```python
from build123d import *

# Parameters (mm, degrees)
F2_DEPTH = 7.5


with BuildPart() as f1:
    # F0 (on Front) → F1 (revolve)
    with BuildSketch(Plane.XZ):
        with BuildLine():
            Line((16.234176, 0), (0, 0))
            Line((0, 0), (0, -18.89116))
            Line((0, -18.89116), (14.934336, -18.89116))
            ThreePointArc((14.934336, -18.89116), (14.908992, -14.946672), (16.234176, -11.231363))
            ThreePointArc((16.234176, -11.231363), (14.748893, -5.615682), (16.234176, 0))
        make_face()
    revolve(axis=Axis((0, 0, -9.44558), (0, 0, 1)))

    # F0 (on Front) → F2 (join, symmetric)
    with BuildSketch(Plane.XZ):
        Polygon((-16.234176, 0), (0, 0), (16.234176, 0), (50.981011, 61.091773), (0, 34.319621), (-50.981011, 61.091773), align=None)
        with BuildLine():
            Line((16.234176, 0), (0, 0))
            Line((0, 0), (0, -18.89116))
            Line((0, -18.89116), (14.934336, -18.89116))
            ThreePointArc((14.934336, -18.89116), (14.908992, -14.946672), (16.234176, -11.231363))
            ThreePointArc((16.234176, -11.231363), (14.748893, -5.615682), (16.234176, 0))
        make_face()
    extrude(amount=F2_DEPTH, both=True)


solid = f1.part
```
Verification items for the finished model (mm, model axes). A direction names the side the tool comes from. Coordinates: 2 decimals unless noted, no trailing zeros. Write each loop counter-clockwise with the first axis right and the second up, starting at its lowest first coordinate (ties: lowest second). Pieces come first, ordered by that corner, then holes. Notation, with made-up numbers: (-39, 4.5) - (-4, 4.5) arc R28 cw to (-4, 30.5) - close; hole circle Ø7 at (26, 19.25). An arc over 180 degrees is marked (long way). Write item = value, one per line.
Q1. Mould release check, pull along Z, two halves, no side actions. Record for faces 1 (the face through (33.364, -0.105, 30.118)), 2 (the face through (25.847, -0.105, 47.893)), 3 (the face through (14.9, -0.1, -15)): released by +Z, released by -Z, zero draft, split by the parting line, or undercut.
Answer:
face_1 = released by -Z
face_2 = released by +Z
face_3 = undercut
Q2. Material ranges on L1, parallel to Y at x = -3, z = 19; L2, parallel to X at y = -3, z = 55; L3, parallel to Z at x = 10.5, y = 8, recorded low to high. Write a range as from..to.
Answer:
L1 = -7.5..7.5
L2 = -47.52..-39.38, 39.38..47.52
L3 = -18.89..0
Q3. Access from +Z, -Z, +X, -X, +Y, -Y to the whole of each face (thin tool, end or side, straight path). Record for faces 4 (the face through (0, 11, 0)), 5 (the face through (0, -11, 0)), 6 (the face through (-25.1, -0.1, 47.5)), 7 (the face through (-33.85, -0.11, 30.97)).
Answer:
face_4 = +Z, +X, -X, +Y
face_5 = +Z, +X, -X, -Y
face_6 = +Z, +Y, -Y
face_7 = -Z, -X, +Y, -Y
Q4. Cross-section at B-B (x = 37). Enter the section's corners in (y, z).
Answer:
outline = (-7.5, 36.51) - (7.5, 36.51) - (7.5, 53.75) - (-7.5, 53.75) - close
Q5. Cross-section at C-C (z = 43.5). Enter the section's corners in (x, y).
Answer:
outline = (-40.98, -7.5) - (-17.48, -7.5) - (-17.48, 7.5) - (-40.98, 7.5) - close; (17.48, -7.5) - (40.98, -7.5) - (40.98, 7.5) - (17.48, 7.5) - close
Q6. Cross-section at A-A (z = 35.5). Enter the section's corners in (x, y), plus the area to 3 significant figures.
Answer:
outline = (-36.43, -7.5) - (-2.25, -7.5) - (-2.25, 7.5) - (-36.43, 7.5) - close; (2.25, -7.5) - (36.43, -7.5) - (36.43, 7.5) - (2.25, 7.5) - close
area = 1,030 mm²
Q7. Cross-section at D-D (z = -13). Enter the section's corners in (x, y).
Answer:
outline = (13.47, -7.5) - (15.42, -7.5) - (15.42, 7.5) - (13.47, 7.5) arc R15.42 ccw (long way) to start
Q8. Go/stop test with flat-tipped pins: pin 1 Ø7 at (x, y) = (5, -11.5) entering from +Z; pin 2 Ø12 at (y, z) = (-2, 0) entering from +X; pin 3 Ø5 at (y, z) = (9, 9.5) entering from +X. Record where each tip stops, or that it passes through.
Answer:
pin_1 = 0
pin_2 = 19.65
pin_3 = 22.77
